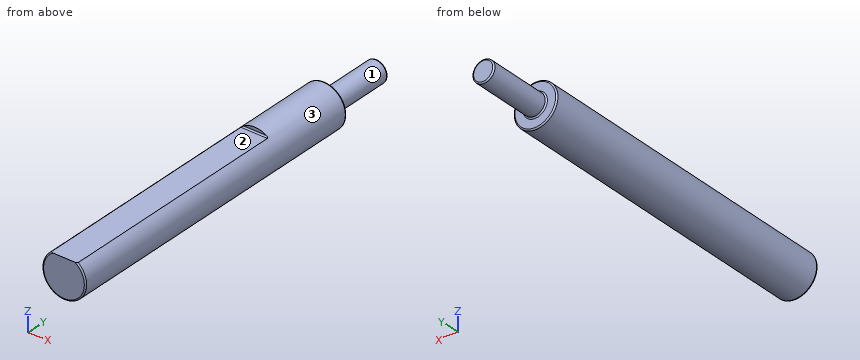
```python
from build123d import *

# Parameters (mm, degrees)
F3_DEPTH = 69.85
F4_R     = 0.381
F5_R     = 0.381
F6_R     = 0.381


with BuildPart() as f1:
    # F0 (on Right) → F1 (revolve)
    with BuildSketch(Plane.YZ):
        Polygon((74.4140613498, 0), (74.4140613498, 3.175), (55.3640613498, 3.175), (55.3640613498, 6.35), (-39.8859386502, 6.35), (-39.8859386502, 0), align=None)
    revolve(axis=Axis((0, 17.2640613498, 0), (0, 1, 0)))

    # F2 (on face) → F3 (cut)
    with BuildSketch(Plane.XZ.offset(39.8859386502)):
        with BuildLine():
            ThreePointArc((3.8766764739, 5.0293020904), (0, 6.35), (-3.8766764739, 5.0293020904))
            Line((-3.8766764739, 5.0293020904), (3.8766764739, 5.0293020904))
        make_face()
    extrude(amount=-F3_DEPTH, mode=Mode.SUBTRACT)

    # F4
    f4_edges = [f1.edges().sort_by_distance(p)[0] for p in [
        (0, 55.364061, -6.35),
        (0, 74.414061, -3.175),
        (0, 55.364061, -3.175),
        (0, 64.889061, 3.175),
    ]]
    fillet(f4_edges, radius=F4_R)

    # F5
    f5_edges = [f1.edges().sort_by_distance(p)[0] for p in [
        (0, -39.885939, -6.35),
    ]]
    fillet(f5_edges, radius=F5_R)

    # F6
    f6_edges = [f1.edges().sort_by_distance(p)[0] for p in [
        (0, 29.964061, 5.029302),
    ]]
    fillet(f6_edges, radius=F6_R)


solid = f1.part
```
Could you check a few things on this model? Use its own coordinates, in mm. Face numbers are marked on the shaded views. A direction names the side the tool comes from. Round coordinates to 2 decimals unless told otherwise and drop trailing zeros. Loops run counter-clockwise (first coordinate to the right, second up) from the corner with the lowest first, then second, coordinate; pieces in that order, holes last.
Q1. I want a section at D-D (y = 58). Write out the boundary of the cut face in (x, z) (3 decimals).
Q2. I want a section at B-B (x = 0). Write out the boundary of the cut face in (y, z) (3 decimals).
Q3. For P1, Ø0.8, axis at x = -0.5, z = 6, coming from the -Y side; P2, Ø1, axis at x = -4, z = 1.5, coming from the +Y side; P3, Ø3, axis at y = 50.5, z = 3.5, coming from the -X side, each with a flat end and sliding along its axis, tell me the tip position at first contact or that it passes through.
Q4. Please list where these lines run through material, in increasing order: L1, parallel to X at y = -10, z = -5.25; L2, parallel to Y at x = 1.25, z = -5; L3, parallel to Y at x = -0.25, z = 5.75.
Q5. On a 3-axis mill with a long thin cutter (end or side, diameter ignored), from which of +Z, -Z, +X, -X, +Y, -Y can I reach the whole of each face in a straight line? I mean the marked faces 1, 2 and 3. Say none if no direction works.
Q6. I want a section at A-A (z = 0). Write out the boundary of the cut face in (x, y) (3 decimals), and give its area (3 significant figures).
Q7. I want a section at C-C (y = 28). Write out the boundary of the cut face in (x, z), and give its area (3 significant figures).
Answer below:
1. outline: circle Ø6.35 at (0, 0)
2. outline: (-39.886, -5.969) arc R0.381 ccw to (-39.505, -6.35) - (54.983, -6.35) arc R0.381 ccw to (55.364, -5.969) - (55.364, -3.556) arc R0.381 cw to (55.745, -3.175) - (74.033, -3.175) arc R0.381 ccw to (74.414, -2.794) - (74.414, 2.794) arc R0.381 ccw to (74.033, 3.175) - (55.745, 3.175) arc R0.381 cw to (55.364, 3.556) - (55.364, 5.969) arc R0.381 ccw to (54.983, 6.35) - (29.964, 6.35) - (29.964, 5.41) arc R0.381 cw to (29.583, 5.029) - (-39.886, 5.029) - close
3. P1: stops at y = 29.96
3. P2: stops at y = 55.36
3. P3: stops at x = -6.03
4. L1: x = -3.57 to 3.57
4. L2: y = -39.89 to 55.36
4. L3: y = 29.96 to 55.36
5. face 1: +Y
5. face 2: +Z, +X, -X, -Y
5. face 3: +Y, -Y
6. outline: (-6.35, -39.505) arc R0.381 ccw to (-5.969, -39.886) - (5.969, -39.886) arc R0.381 ccw to (6.35, -39.505) - (6.35, 54.983) arc R0.381 ccw to (5.969, 55.364) - (3.556, 55.364) arc R0.381 cw to (3.175, 55.745) - (3.175, 74.033) arc R0.381 ccw to (2.794, 74.414) - (-2.794, 74.414) arc R0.381 ccw to (-3.175, 74.033) - (-3.175, 55.745) arc R0.381 cw to (-3.556, 55.364) - (-5.969, 55.364) arc R0.381 ccw to (-6.35, 54.983) - close
6. area: 1,330 mm2
7. outline: (-3.88, 5.03) arc R6.35 ccw (long way) to (3.88, 5.03) - close
7. area: 120 mm2
